```python
from build123d import *

# Parameters (mm, degrees)
SKETCH1_W                = 37.8
SKETCH1_H                = 16.2
RETAINER_PLATE_DEPTH     = 2
SKETCH2_W                = 18
SKETCH2_H                = 7.5
RIBBON_SLOT_DEPTH        = 4
SKETCH3_R                = 1.2
M2_CLEARANCE_HOLES_DEPTH = 4


with BuildPart() as part:
    # Sketch1 → Retainer Plate (new body)
    with BuildSketch(Plane(origin=(0, 15, 0), x_dir=(1, 0, 0), z_dir=(0, 1, 0))):
        with Locations((0, 37.4)):
            Rectangle(SKETCH1_W, SKETCH1_H)
    extrude(amount=RETAINER_PLATE_DEPTH)

    # Sketch2 → Ribbon Slot (cut)
    with BuildSketch(Plane(origin=(0, 14, 0), x_dir=(1, 0, 0), z_dir=(0, 1, 0))):
        with Locations((0, 35.2)):
            Rectangle(SKETCH2_W, SKETCH2_H)
    extrude(amount=RIBBON_SLOT_DEPTH, mode=Mode.SUBTRACT)

    # Sketch3 → M2 Clearance Holes (cut)
    with BuildSketch(Plane(origin=(0, 14, 0), x_dir=(1, 0, 0), z_dir=(0, 1, 0))):
        with Locations(Location((-16.9, 31, 0), (0, 0, 270))):
            Circle(SKETCH3_R)
        with Locations(Location((-16.9, 43.5, 0), (0, 0, 270))):
            Circle(SKETCH3_R)
        with Locations(Location((16.9, 31, 0), (0, 0, 270))):
            Circle(SKETCH3_R)
        with Locations(Location((16.9, 43.5, 0), (0, 0, 270))):
            Circle(SKETCH3_R)
    extrude(amount=M2_CLEARANCE_HOLES_DEPTH, mode=Mode.SUBTRACT)


solid = part.part
```
The listing builds one solid part. Answer for the finished solid, in the listing's coordinates (mm). A direction names the side the tool comes from. Coordinates: 2 decimals unless noted, no trailing zeros. Order: outer loops, then holes, each group sorted by start corner. A loop starts at its lowest first (then second) coordinate and runs counter-clockwise, first axis right, second up. Notation, with made-up numbers: M 64,9 L 79,9 A7 cw 79,16 Z; hole C 9,-29 d2. An arc over 180 degrees is marked long. Answer as a JSON object with one key per item and string values. Group by question number.
1. Determine the mould class of faces 3 (the flat face through (0, 16, -29.3)), 4 (the flat face through (0, 16, -38.95)), 5 (the cylindrical face through (-15.89, 15.99, -30.35)), 6 (the flat face through (-0.3, 17, -39.3)) for opening direction Z: released by +Z, released by -Z, zero draft, split by the parting line, or undercut.
2. Section D-D on x = 16.9 is taken. Write down the section's boundary in (y, z).
3. Section C-C on y = 15.5 is taken. Write down the section's boundary in (x, z), then the cut area to 3 significant figures.
4. Straight lines are drawn through the part: line 1 (Z direction, x = 16.9, y = 16.45); line 2 (X direction, y = 16.5, z = -31); line 3 (Z direction, x = 6, y = 15.4). For each, find the intervals that lie inside material, in ascending order.
5. Section B-B on z = -43.5 is taken. Write down the section's boundary in (x, y), then the cut area to 3 significant figures.
6. Section A-A on z = -37.25 is taken. Write down the section's boundary in (x, y), then the cut area to 3 significant figures.
7. A tool of negligible diameter and unlimited length cuts with its end or side. For faces 1 (the flat face through (9, 16, -35)), 2 (the flat face through (-18.9, 16, -37)), from which of +Z, -Z, +X, -X, +Y, -Y can it reach the whole face along a straight path? Write none if from no direction.
Values follow:
{
 "1": {"face 3": "released by +Z", "face 4": "undercut", "face 5": "undercut", "face 6": "zero draft"},
 "2": {"outline": "M 15,-45.5 L 17,-45.5 L 17,-44.7 L 15,-44.7 Z; M 15,-42.3 L 17,-42.3 L 17,-32.2 L 15,-32.2 Z; M 15,-29.8 L 17,-29.8 L 17,-29.3 L 15,-29.3 Z"},
 "3": {"outline": "M -18.9,-45.5 L 18.9,-45.5 L 18.9,-29.3 L -18.9,-29.3 Z; hole C -16.9,-43.5 d2.4; hole C -16.9,-31 d2.4; hole M -9,-38.95 L 9,-38.95 L 9,-31.45 L -9,-31.45 Z; hole C 16.9,-43.5 d2.4; hole C 16.9,-31 d2.4", "area": "459 mm2"},
 "4": {"line 1": "-45.5 to -44.7, -42.3 to -32.2, -29.8 to -29.3", "line 2": "-18.9 to -18.1, -15.7 to 15.7, 18.1 to 18.9", "line 3": "-45.5 to -38.95, -31.45 to -29.3"},
 "5": {"outline": "M -18.9,15 L -18.1,15 L -18.1,17 L -18.9,17 Z; M -15.7,15 L 15.7,15 L 15.7,17 L -15.7,17 Z; M 18.1,15 L 18.9,15 L 18.9,17 L 18.1,17 Z", "area": "66.0 mm2"},
 "6": {"outline": "M -18.9,15 L -9,15 L -9,17 L -18.9,17 Z; M 9,15 L 18.9,15 L 18.9,17 L 9,17 Z", "area": "39.6 mm2"},
 "7": {"face 1": "+Y, -Y", "face 2": "+Z, -Z, -X, +Y, -Y"}
}
